Autodesk Inventor part; units mm, degrees
ref_plane "Work Plane2" through (0, 0, -6.75) normal (0, 0, 1) x (1, 0, 0)
ref_plane "YZ Plane" through (0, 0, 0) normal (1, 0, 0) x (0, 1, 0)
ref_plane "XZ Plane" through (0, 0, 0) normal (0, 1, 0) x (-1, 0, 0)
sketch "Sketch1" plane through (0, 0, 0) normal (0, 1, 0) x (-1, 0, 0)
  line L0 (5.75, 3.75) -> (-5.75, 3.75)
  line L1 (-5.75, 3.75) -> (-5.75, -3.75)
  line L2 (-5.75, -3.75) -> (5.75, -3.75)
  line L3 (5.75, -3.75) -> (5.75, 3.75)
  line L4 (5.75, 3.75) -> (-5.75, -3.75) construction
  line L5 (-5.75, 3.75) -> (5.75, -3.75) construction
  line L6 (0, 0) -> (0, 3.75)
  circle A0 centre (10, 0.5) radius 1.25
  circle A1 centre (-10, 0.5) radius 1.25
  line L7 (8.328, 1.75) -> (12.3503, 1.75)
  line L8 (8.75, 3.0207) -> (8.75, -2.5964)
  line L9 (5.05, 3.25) -> (-5.05, 3.25)
  line L10 (-5.05, 3.25) -> (-5.05, -3.25)
  line L11 (-5.05, -3.25) -> (5.05, -3.25)
  line L12 (5.05, -3.25) -> (5.05, 3.25)
  line L13 (5.05, 3.25) -> (-5.05, -3.25) construction
  line L14 (-5.05, 3.25) -> (5.05, -3.25) construction
  dimension "d7" = 2.5
  dimension "d13" = 7.5
  dimension "d14" = 11.5
  dimension "d16" = 2
  dimension "d17" = 3
  dimension "d31" = 10.1
  dimension "d32" = 6.5
sketch "Sketch2" plane through (0, 0, 0) normal (0, 0, 1) x (1, 0, 0)
  line L0 (0, 0) -> (0, 5)
  line L1 (0, 5) -> (0, 11.5)
  line L2 (-14.9, 5) -> (14.9, 5)
  line L3 (14.9, 5) -> (14.9, 18)
  line L4 (14.9, 18) -> (-14.9, 18)
  line L5 (-14.9, 18) -> (-14.9, 5)
  line L6 (-14.9, 5) -> (14.9, 18) construction
  line L7 (14.9, 5) -> (-14.9, 18) construction
  line L8 (0, 11.5) -> (-18.5, 11.5)
  circle A0 centre (-18.5, 11.5) radius 1.6
  circle A1 centre (18.5, 11.5) radius 1.6
  dimension "d23" = 5
  dimension "d24" = 6.5
  dimension "d25" = 29.8
  dimension "d26" = 13
  dimension "d27" = 18.5
  dimension "d28" = 3.2
ref_plane "Work Plane2" through (0, 0, -6.75) normal (0, 0, 1) x (1, 0, 0)
sketch "Sketch3" plane through (0, 0, -6.75) normal (0, 0, 1) x (1, 0, 0)
  line L0 (0, 0) -> (0, 5)
  line L1 (-14.9, 5) -> (14.9, 5)
  line L2 (-14.9, 18) -> (-14.9, 5)
  line L3 (0, 5) -> (0, 11.5)
  line L4 (0, 11.5) -> (-18.5, 11.5)
  circle A0 centre (-18.5, 11.5) radius 1.6
  line L5 (14.9, 18) -> (-14.9, 18)
  line L6 (14.9, 5) -> (14.9, 18)
  circle A1 centre (18.5, 11.5) radius 1.6
sketch "Sketch4" plane through (0, 0, 0) normal (0, 1, 0) x (-1, 0, 0)
  line L0 (-14.25, -2.75) -> (-5.75, -2.75)
  line L1 (-5.75, -2.75) -> (-5.75, 3.75)
  line L2 (-5.75, 3.75) -> (-14.25, 3.75)
  line L3 (-14.25, 3.75) -> (-14.25, -2.75)
  line L4 (-14.25, -2.75) -> (-5.75, 3.75) construction
  line L5 (-5.75, -2.75) -> (-14.25, 3.75) construction
  line L6 (0, 0) -> (0, 3.75)
  line L7 (14.25, -2.75) -> (5.75, -2.75)
  line L8 (5.75, -2.75) -> (5.75, 3.75)
  line L9 (5.75, 3.75) -> (14.25, 3.75)
  line L10 (14.25, 3.75) -> (14.25, -2.75)
  point P0 (-10, 0.5)
  point P1 (-10, 0.5)
  point P2 (-10, 0.5)
  point P3 (10, 0.5)
  point P4 (10, 0.5)
extrude "Extrusion1" add sketch "Sketch4" along normal blind 2.5 contours L3 L2 L1 L0
extrude "Extrusion2" add sketch "Sketch4" along normal blind 2.5 contours L7 L8 L9 L10
hole "Hole1" at (10, 0, 0.5) at (-10, 0, 0.5) direction (0, 1, 0) diameter 2.8 end through all
sketch "Sketch5" plane through (0, 2.5, 0) normal (0, 1, 0) x (1, 0, 0)
  line L0 (5.75, -3.75) -> (5.75, 2.75)
  line L1 (5.75, 2.75) -> (14.25, 2.75)
  line L2 (14.25, 2.75) -> (14.25, -3.75)
  line L3 (14.25, -3.75) -> (5.75, -3.75)
  line L4 (7.5, 1.85) -> (12.5, 1.85)
  line L5 (12.5, 1.85) -> (12.5, -2.85)
  line L6 (12.5, -2.85) -> (7.5, -2.85)
  line L7 (7.5, -2.85) -> (7.5, 1.85)
  line L8 (0, 0) -> (0, -3.75)
  line L9 (-5.75, -3.75) -> (-5.75, 2.75)
  line L10 (-5.75, 2.75) -> (-14.25, 2.75)
  line L11 (-14.25, 2.75) -> (-14.25, -3.75)
  line L12 (-14.25, -3.75) -> (-5.75, -3.75)
  line L13 (-7.5, 1.85) -> (-12.5, 1.85)
  line L14 (-12.5, 1.85) -> (-12.5, -2.85)
  line L15 (-12.5, -2.85) -> (-7.5, -2.85)
  line L16 (-7.5, -2.85) -> (-7.5, 1.85)
  dimension "d69" = 1.75
  dimension "d70" = 0.9
  dimension "d71" = 1.75
  dimension "d72" = 0.9
extrude "Extrusion8" add sketch "Sketch5" along normal blind 2.5
sketch "Sketch8" plane through (14.25, 0, -2.75) normal (0, 0, -1) x (-1, 0, 0)
  line L0 (14.25, 0) -> (14.25, 5)
  line L1 (8.5, 0) -> (8.5, 5)
  line L2 (0, 5) -> (8.5, 5)
  line L3 (8.5, 5) -> (8.5, 0)
  line L4 (8.5, 0) -> (0, 0)
  line L5 (0, 0) -> (0, 5)
  line L6 (20, 0) -> (20, 5)
  line L7 (28.5, 5) -> (20, 5)
  line L8 (20, 5) -> (20, 0)
  line L9 (20, 0) -> (28.5, 0)
  line L10 (28.5, 0) -> (28.5, 5)
extrude "Extrusion9" add sketch "Sketch8" along normal blind 5
sketch "Sketch10" plane through (14.25, 0, -7.75) normal (0, 0, -1) x (-1, 0, 0)
  line L0 (14.25, 0) -> (14.25, 5)
  line L1 (8.5, 0) -> (-7.5, 0)
  line L2 (8.5, 0) -> (24.5, 0) construction
  line L3 (-7.5, 0) -> (-7.5, 15)
  line L4 (-7.5, 15) -> (-1, 15)
  line L5 (8.5, 0) -> (8.5, 5)
  line L6 (8.5, 5) -> (-1, 5)
  line L7 (-1, 5) -> (-1, 15)
  line L8 (20, 0) -> (36, 0)
  line L9 (36, 0) -> (36, 15)
  line L10 (36, 15) -> (29.5, 15)
  line L11 (20, 0) -> (20, 5)
  line L12 (20, 5) -> (29.5, 5)
  line L13 (29.5, 5) -> (29.5, 15)
  line L14 (8.5, 5) -> (20, 5)
  line L15 (20, 0) -> (8.5, 0)
  point P0 (-4.25, 11.5)
  point P1 (-4.25, 11.5)
  point P2 (32.75, 11.5)
  point P3 (32.75, 11.5)
  dimension "d95" = 16
  dimension "d97" = 15
  dimension "d98" = 6.5
  dimension "d99" = 5
extrude "Extrusion10" add sketch "Sketch10" along normal blind 2.5
hole "Hole2" at (18.5, 11.5, -7.75) at (-18.5, 11.5, -7.75) direction (0, 0, -1) diameter 3.3 end through all
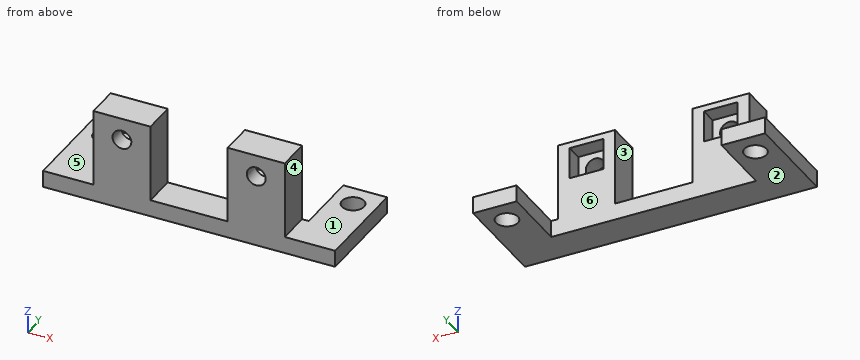
Geometry check sheet. Reference: the model listing, model coordinates, mm. Face numbers are marked on the shaded views. A direction names the side the tool comes from. Round coordinates to 2 decimals unless told otherwise and drop trailing zeros. Order: outer loops, then holes, each group sorted by start corner. A loop starts at its lowest first (then second) coordinate and runs counter-clockwise, first axis right, second up. Notation, with made-up numbers: (74.25, -2) -> (95.25, -2) arc R6 ccw to (95.25, 2) -> close; hole circle Ø3 at (70, 43.5). An arc over 180 degrees is marked (long way). Return JSON: item names as keys, results as strings. Group by question number.
Q1. Material ranges on probe 1 along X at (y, z) = (4.75, 0.5); probe 2 along X at (y, z) = (1.1, 0.5); probe 3 along Z at (x, y) = (10, 1.25), recorded low to high. Write a range as from..to.
Q2. Section check B-B, the plane z = 0.5. Record the boundary of the cut face in (x, y), plus the area to 3 significant figures.
Q3. Release check for a two-part mould opening along X. For the marked faces 4, 5 and 6 record: released by +X, released by -X, zero draft, split by the parting line, or undercut.
Q4. Section check D-D, the plane z = -6.75. Record the boundary of the cut face in (x, y).
Q5. Section check A-A, the plane x = -10. Record the boundary of the cut face in (y, z), plus the area to 4 significant figures.
Q6. Gauge pin test, flat ends, axial feed: pin 1 (3 mm diameter, centred on y = 3.5, z = -0.5, fed in from -X); pin 2 (3 mm diameter, centred on x = -15.5, y = 7.5, fed in from +Z); pin 3 (4.5 mm diameter, centred on x = -10, z = 0.5, fed in from +Y). Record the tip position at first contact, or that the pin passes through.
Q7. Section check C-C, the plane y = 11.5. Record the boundary of the cut face in (x, z).
Q8. Tool access check on the marked faces 1, 2 and 3. Record the directions out of +Z, -Z, +X, -X, +Y, -Y that give a thin tool (end or side, any length) a straight path to the whole face; none if there is none.
Numbers:
{
 "1": {"probe 1": "-14.25..-12.5, -7.5..-5.75, 5.75..7.5, 12.5..14.25", "probe 2": "-14.25..-11.4, -8.6..-5.75, 5.75..8.6, 11.4..14.25", "probe 3": "-10.25..-0.9, 1.9..3.75"},
 "2": {"outline": "(-14.25, 0) -> (-11.4, 0) -> (-11.4, 2.5) -> (-12.5, 2.5) -> (-12.5, 5) -> (-14.25, 5) -> close; (-8.6, 0) -> (-5.75, 0) -> (-5.75, 5) -> (-7.5, 5) -> (-7.5, 2.5) -> (-8.6, 2.5) -> close; (5.75, 0) -> (8.6, 0) -> (8.6, 2.5) -> (7.5, 2.5) -> (7.5, 5) -> (5.75, 5) -> close; (11.4, 0) -> (14.25, 0) -> (14.25, 5) -> (12.5, 5) -> (12.5, 2.5) -> (11.4, 2.5) -> close", "area": "46.0 mm^2"},
 "3": {"face 4": "released by +X", "face 5": "zero draft", "face 6": "undercut"},
 "4": {"outline": "(-14.25, 0) -> (-5.75, 0) -> (-5.75, 5) -> (-14.25, 5) -> close; (5.75, 0) -> (14.25, 0) -> (14.25, 5) -> (5.75, 5) -> close"},
 "5": {"outline": "(0, -10.25) -> (5, -10.25) -> (5, -1.85) -> (2.5, -1.85) -> (2.5, -0.9) -> (0, -0.9) -> close; (0, 1.9) -> (2.5, 1.9) -> (2.5, 2.85) -> (5, 2.85) -> (5, 3.75) -> (0, 3.75) -> close", "area": "51.25 mm^2"},
 "6": {"pin 1": "x = -14.25", "pin 2": "z = -7.75", "pin 3": "y = 2.5"},
 "7": {"outline": "(-21.75, -10.25) -> (-20.15, -10.25) -> (-20.15, -7.75) -> (-21.75, -7.75) -> close; (-16.85, -10.25) -> (-15.25, -10.25) -> (-15.25, -7.75) -> (-16.85, -7.75) -> close; (15.25, -10.25) -> (16.85, -10.25) -> (16.85, -7.75) -> (15.25, -7.75) -> close; (20.15, -10.25) -> (21.75, -10.25) -> (21.75, -7.75) -> (20.15, -7.75) -> close"},
 "8": {"face 1": "+Z, +X, +Y, -Y", "face 2": "-Z, +X, -X, +Y, -Y", "face 3": "+Z, +Y, -Y"}
}
